Read the model definition and answer for the solid it produces. Units are mm, in the model's axes. Face numbers are marked on the shaded views. A direction names the side the tool comes from. Coordinates: 2 decimals unless noted, no trailing zeros. Loops run counter-clockwise (first coordinate to the right, second up) from the corner with the lowest first, then second, coordinate; pieces in that order, holes last. Notation, with made-up numbers: (21, 79) -> (33, 79) arc R25 ccw to (33, 109) -> close; hole circle Ø9 at (19.5, -18). An arc over 180 degrees is marked (long way). One line per question, with ' | ' between items. Start each with the question number.
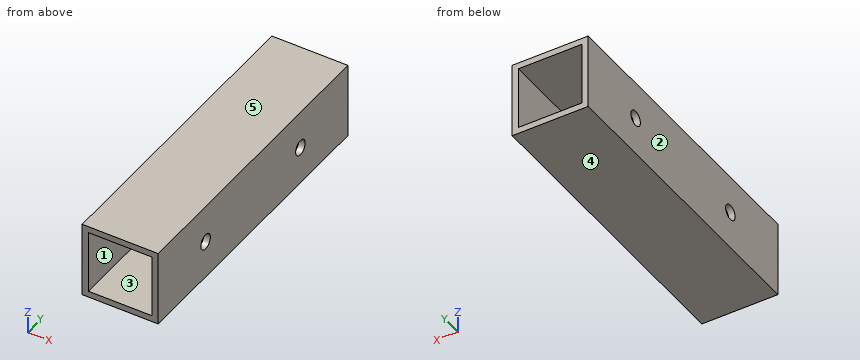
```python
from build123d import *

# Parameters (mm, degrees)
SKETCH1_W           = 38.1
SKETCH1_H           = 38.1
SKETCH1_W_2         = 31.75
SKETCH1_H_2         = 31.75
BOSS_EXTRUDE1_DEPTH = 152.4
SKETCH2_R           = 3.81
CUT_EXTRUDE1_DEPTH  = 152.4


with BuildPart() as part:
    # Sketch1 → Boss-Extrude1 (new body)
    with BuildSketch(Plane(origin=(0, 0, 0), x_dir=(1, 0, 0), z_dir=(0, 1, 0))):
        Rectangle(SKETCH1_W, SKETCH1_H)
        Rectangle(SKETCH1_W_2, SKETCH1_H_2, mode=Mode.SUBTRACT)
    extrude(amount=BOSS_EXTRUDE1_DEPTH)

    # Sketch2 → Cut-Extrude1 (cut)
    with BuildSketch(Plane.ZY.offset(19.05)):
        with Locations((0, 114.3)):
            Circle(SKETCH2_R)
        with Locations((0, 38.1)):
            Circle(SKETCH2_R)
    extrude(amount=-CUT_EXTRUDE1_DEPTH, mode=Mode.SUBTRACT)


solid = part.part
```
(1) Determine the mould class of the marked faces 3, 4 and 5 for opening direction Z: +Z half, -Z half, draft (parallel to the pull), parting line (faces both ways), or undercut.
(2) Section B-B on x = 3.5 is taken. Write down the section's boundary in (y, z) (3 decimals).
(3) Section D-D on z = -10.5 is taken. Write down the section's boundary in (x, y) (3 decimals).
(4) Find the intervals of material crossed by probe 1 along Y at (x, z) = (17.2, 0); probe 2 along X at (y, z) = (30, -13) (3 decimals), in increasing order. Write a range as from..to.
(5) Section A-A on z = 0 is taken. Write down the section's boundary in (x, y) (3 decimals).
(6) A tool of negligible diameter and unlimited length cuts with its end or side. For the marked faces 1 and 2, from which of +Z, -Z, +X, -X, +Y, -Y can it reach the whole face along a straight path? Write none if from no direction.
(7) Section C-C on y = 38.1 is taken. Write down the section's boundary in (x, z) (3 decimals), plus the area to 3 significant figures.
Working result:
1) face 3: undercut | face 4: -Z half | face 5: +Z half
2) outline: (0, -19.05) -> (152.4, -19.05) -> (152.4, -15.875) -> (0, -15.875) -> close; (0, 15.875) -> (152.4, 15.875) -> (152.4, 19.05) -> (0, 19.05) -> close
3) outline: (-19.05, 0) -> (-15.875, 0) -> (-15.875, 152.4) -> (-19.05, 152.4) -> close; (15.875, 0) -> (19.05, 0) -> (19.05, 152.4) -> (15.875, 152.4) -> close
4) probe 1: y = 0..34.29, 41.91..110.49, 118.11..152.4 | probe 2: x = -19.05..-15.875, 15.875..19.05
5) outline: (-19.05, 0) -> (-15.875, 0) -> (-15.875, 34.29) -> (-19.05, 34.29) -> close; (-19.05, 41.91) -> (-15.875, 41.91) -> (-15.875, 110.49) -> (-19.05, 110.49) -> close; (-19.05, 118.11) -> (-15.875, 118.11) -> (-15.875, 152.4) -> (-19.05, 152.4) -> close; (15.875, 0) -> (19.05, 0) -> (19.05, 34.29) -> (15.875, 34.29) -> close; (15.875, 41.91) -> (19.05, 41.91) -> (19.05, 110.49) -> (15.875, 110.49) -> close; (15.875, 118.11) -> (19.05, 118.11) -> (19.05, 152.4) -> (15.875, 152.4) -> close
6) face 1: +Y, -Y | face 2: +Z, -Z, -X, +Y, -Y
7) outline: (-19.05, -19.05) -> (19.05, -19.05) -> (19.05, -3.81) -> (15.875, -3.81) -> (15.875, -15.875) -> (-15.875, -15.875) -> (-15.875, -3.81) -> (-19.05, -3.81) -> close; (-19.05, 3.81) -> (-15.875, 3.81) -> (-15.875, 15.875) -> (15.875, 15.875) -> (15.875, 3.81) -> (19.05, 3.81) -> (19.05, 19.05) -> (-19.05, 19.05) -> close | area: 395 mm2
